```python
from build123d import *

# Parameters (mm, degrees)
BOX002_W               = 55
BOX002_H               = 100
BOX002_DEPTH           = 10
SKETCH010_W            = 75
SKETCH010_H            = 120
PAD009_DEPTH           = 10
CUT037_ROLL_ANGLE      = 5e-06
CUT037_PITCH_ANGLE     = 53.219477
CUT037_PLACEMENT_ANGLE = 9e-06


with BuildPart() as box002:
    # Box002 → Box002 (new body)
    with BuildSketch(Plane(origin=(-115, 45.8, 7.5), x_dir=(1, 0, 0), z_dir=(0, 0, 1))):
        with Locations((27.5, 50)):
            Rectangle(BOX002_W, BOX002_H)
    extrude(amount=BOX002_DEPTH)


with BuildPart() as display:
    # Sketch010 → Pad009 (new body)
    with BuildSketch(Plane.XY):
        with Locations((-87.509099, 96.743134)):
            Rectangle(SKETCH010_W, SKETCH010_H)
    extrude(amount=PAD009_DEPTH)

    # Cut037: cut Box002
    add(box002.part, mode=Mode.SUBTRACT)


with BuildPart() as display_1:
    # Cut037 roll: moved
    add(display.part.rotate(Axis((0, 0, 0), (1, 0, 0)), CUT037_ROLL_ANGLE))


with BuildPart() as display_2:
    # Cut037 pitch: moved
    add(display_1.part.rotate(Axis((0, 0, 0), (0, 1, 0)), CUT037_PITCH_ANGLE))


with BuildPart() as display_3:
    # Cut037 placement: moved
    add(display_2.part.moved(Location((-34.792314, -97.00353, 121.476113))).rotate(Axis((-34.792314, -97.00353, 121.476113), (0, 0, 1)), CUT037_PLACEMENT_ANGLE))


solid = display_3.part
```
Source: CAD feature listing. Evaluate the final solid. Frame: model axes, mm. Round coordinates to 2 decimals unless told otherwise and drop trailing zeros. Write each loop counter-clockwise with the first axis right and the second up, starting at its lowest first coordinate (ties: lowest second). Pieces come first, ordered by that corner, then holes. Notation, with made-up numbers: M -38,28.25 L 16,28.25 A18 ccw 16,45.25 Z; hole C -4.5,49.25 d5. An arc over 180 degrees is marked long. Answer as a JSON object with one key per item and string values. Group by question number.
(1) Section query D-D on x = -60.5. Output: boundary loops of the cut face in (y, z).
(2) Section query A-A on y = -8. Output: boundary loops of the cut face in (x, z).
(3) First-contact query: pin 1 (4 mm diameter, centred on x = -67.5, y = -11.5, fed in from -Z); pin 2 (2 mm diameter, centred on y = 39, z = 176, fed in from -X); pin 3 (2 mm diameter, centred on y = -33, z = 198, fed in from +X). Flat tips, straight axial feed; report the tip coordinate or a pass-through.
(4) Section query B-B on x = -68. Output: boundary loops of the cut face in (y, z), then the cut area to 3 significant figures.
(5) Section query C-C on z = 169. Output: boundary loops of the cut face in (x, y).
(6) Mould query, pull axis Y, two halves, no side actions, for faces 1 (the flat face through (-105.693, -1.1, 224.552)), 2 (the flat face through (-80, -51.204, 197)), 3 (the flat face through (-84, 59.74, 195)). Classes: +Y half, -Y half, draft (parallel to the pull), parting line (faces both ways), or undercut.
(7) Ray query, line 1 (X direction, y = -1.5, z = 220); line 2 (Z direction, x = -105, y = 54.5); line 3 (X direction, y = 3, z = 207.5). Return the intervals inside material, ascending. Write a range as [from, to].
Computed values:
{
 "1": {"outline": "M -60.26,164.7 L 59.74,164.7 L 59.74,172.57 L -60.26,172.57 Z"},
 "2": {"outline": "M -109.64,221.6 L -64.74,161.53 L -56.73,167.52 L -62.71,175.52 L -64.71,174.02 L -97.64,218.07 L -95.64,219.57 L -101.63,227.59 Z"},
 "3": {"pin 1": "z = 162.55", "pin 2": "x = -76.3", "pin 3": "x = -81.89"},
 "4": {"outline": "M -60.26,165.9 L 59.74,165.9 L 59.74,182.6 L 48.8,182.6 L 48.8,178.42 L -51.2,178.42 L -51.2,182.6 L -60.26,182.6 Z", "area": "1,590 mm^2"},
 "5": {"outline": "M -70.32,-60.26 L -57.83,-60.26 L -57.83,59.74 L -70.32,59.74 Z"},
 "6": {"face 1": "draft", "face 2": "undercut", "face 3": "+Y half"},
 "7": {"line 1": "[-108.45, -95.96]", "line 2": "[215.39, 225.07]", "line 3": "[-99.1, -89.74]"}
}
